```python
from build123d import *

# Parameters (mm, degrees)
SKETCH1_W           = 127
SKETCH1_H           = 38.1
BOSS_EXTRUDE1_DEPTH = 132.08
CUT_EXTRUDE1_DEPTH  = 35.56
BOSS_EXTRUDE2_DEPTH = 2.54
BOSS_EXTRUDE3_START = 127
BOSS_EXTRUDE3_DEPTH = 2.54
SKETCH4_R           = 3.175
CUT_EXTRUDE2_DEPTH  = 2.54


with BuildPart() as part:
    # Sketch1 → Boss-Extrude1 (new body)
    with BuildSketch(Plane.XY):
        with Locations((63.5, 19.05)):
            Rectangle(SKETCH1_W, SKETCH1_H)
    extrude(amount=BOSS_EXTRUDE1_DEPTH)

    # Sketch2 → Cut-Extrude1 (cut)
    with BuildSketch(Plane(origin=(0, 38.1, 0), x_dir=(1, 0, 0), z_dir=(0, 1, 0))):
        Polygon((0, -25.4), (2.54, -25.4), (2.54, -132.08), (124.46, -132.08), (124.46, -25.4), (127, -25.4), (127, 0), (0, 0), align=None)
    extrude(amount=-CUT_EXTRUDE1_DEPTH, mode=Mode.SUBTRACT)

    # Sketch3 → Boss-Extrude2 (add)
    with BuildSketch(Plane(origin=(0, 0, 0), x_dir=(0, 0, -1), z_dir=(1, 0, 0))):
        Polygon((-25.4, 2.54), (-14.986, 38.1), (-25.4, 38.1), align=None)
    extrude(amount=BOSS_EXTRUDE2_DEPTH)

    # Sketch3<2> → Boss-Extrude3 (add)
    with BuildSketch(Plane(origin=(0, 0, 0), x_dir=(0, 0, -1), z_dir=(1, 0, 0)).offset(BOSS_EXTRUDE3_START)):
        Polygon((-25.4, 2.54), (-14.986, 38.1), (-25.4, 38.1), align=None)
    extrude(amount=-BOSS_EXTRUDE3_DEPTH)

    # Sketch4 → Cut-Extrude2 (cut)
    with BuildSketch(Plane(origin=(0, 2.54, 0), x_dir=(1, 0, 0), z_dir=(0, 1, 0))):
        with Locations(Location((31.75, -12.7, 0), (0, 0, 180))):
            Circle(SKETCH4_R)
        with Locations(Location((95.25, -12.7, 0), (0, 0, 180))):
            Circle(SKETCH4_R)
    extrude(amount=-CUT_EXTRUDE2_DEPTH, mode=Mode.SUBTRACT)


solid = part.part
```
Geometry: final body of the model. Coordinates: model frame, mm. A direction names the side the tool comes from. Give positions to 0.01 mm unless a question says otherwise; leave off trailing zeros. Loops run counter-clockwise (first coordinate to the right, second up) from the corner with the lowest first, then second, coordinate; pieces in that order, holes last. Notation, with made-up numbers: (31.25, 16.25) -> (44.25, 16.25) arc R24 cw to (44.25, 40.25) -> close; hole circle Ø5 at (18, 53.5). An arc over 180 degrees is marked (long way). Use one line per item in the form item = value.
Item 1: Section query B-B on y = 27. Output: boundary loops of the cut face in (x, z), and give its area (3 significant figures).
A:
outline = (0, 18.24) -> (2.54, 18.24) -> (2.54, 132.08) -> (0, 132.08) -> close; (124.46, 18.24) -> (127, 18.24) -> (127, 132.08) -> (124.46, 132.08) -> close
area = 578 mm^2
Item 2: Section query C-C on z = 72. Output: boundary loops of the cut face in (x, y), and give its area (3 significant figures).
A:
outline = (0, 0) -> (127, 0) -> (127, 38.1) -> (124.46, 38.1) -> (124.46, 2.54) -> (2.54, 2.54) -> (2.54, 38.1) -> (0, 38.1) -> close
area = 503 mm^2
Item 3: Pin query (flat end, axial travel): P1, Ø1, axis at x = 114, z = 57.5, coming from the +Y side. Return the tip coordinate at first contact, or that it passes through.
A:
P1 = 2.54
Item 4: Line query: probe 1 along Z at (x, y) = (31.75, 0.85) (3 decimals); probe 2 along X at (y, z) = (1, 12); probe 3 along X at (y, z) = (33, 48). Output: solid intervals per line, ascending.
A:
probe_1 = 0 to 9.525, 15.875 to 132.08
probe_2 = 0 to 28.65, 34.85 to 92.15, 98.35 to 127
probe_3 = 0 to 2.54, 124.46 to 127
Item 5: Section query A-A on x = 31.75. Output: boundary loops of the cut face in (y, z) (3 decimals), and give its area (3 significant figures).
A:
outline = (0, 0) -> (2.54, 0) -> (2.54, 9.525) -> (0, 9.525) -> close; (0, 15.875) -> (2.54, 15.875) -> (2.54, 132.08) -> (0, 132.08) -> close
area = 319 mm^2
Item 6: Draft query along Y for faces 1 (the face through (63, 0, 65)), 2 (the face through (125.748, 20.071, 20.266)), 3 (the face through (2.54, 21, 74)), 4 (the face through (1.252, 20.071, 20.266)). Return one class per face: pulls with the +Y half, pulls with the -Y half, needs draft (parallel to the pull), parting line crosses it, or undercut.
A:
face_1 = pulls with the -Y half
face_2 = undercut
face_3 = needs draft
face_4 = undercut
Item 7: Access query for faces 5 (the face through (34.92, 1.29, 12.84)), 6 (the face through (124.46, 21, 74)). Directions: +Z, -Z, +X, -X, +Y, -Y. A direction counts if a zero-diameter tool reaches every point of the face in a straight line with its end or side. Return the directions, or none.
A:
face_5 = +Y, -Y
face_6 = +Z, -Z, +Y
